Geometry: final body of the model. Coordinates: model frame, mm. Face numbers are marked on the shaded views. A direction names the side the tool comes from. Give positions to 0.01 mm unless a question says otherwise; leave off trailing zeros. Order: outer loops, then holes, each group sorted by start corner. A loop starts at its lowest first (then second) coordinate and runs counter-clockwise, first axis right, second up. Notation, with made-up numbers: (29.5, 49) - (73.5, 49) arc R17 cw to (73.5, 56) - close; hole circle Ø8 at (30, 88). An arc over 180 degrees is marked (long way). Put each result on its own line as item: value. Start each with the question number.
1. Ray query, line 1 along X through (y, z) = (-22, 3); line 2 along Y through (x, z) = (-36.5, 21); line 3 along X through (y, z) = (-43, 10). Return the intervals inside material, ascending. Write a range as from..to.
2. First-contact query: P1, Ø11, axis at y = -72, z = 28.5, coming from the +X side; P2, Ø1.5, axis at y = -9, z = 6, coming from the +X side; P3, Ø13.5, axis at x = -40, y = -15, coming from the +Z side. Flat tips, straight axial feed; report the tip coordinate or a pass-through.
3. Section B-B on x = -52.5. Return the cut outline in (y, z), plus the area to 3 significant figures.
4. Section D-D on y = -32.5. Return the cut outline in (x, z), plus the area to 3 significant figures.
5. Section C-C on z = 5. Return the cut outline in (x, y), plus the area to 3 significant figures.
6. Set-up query: the marked faces 1, 2 and 3. Return all of +Z, -Z, +X, -X, +Y, -Y with unobstructed straight access to the full face (end or side cutting, diameter ignored); none if empty.
7. Mould query, pull axis Y, two halves, no side actions, for the marked faces 4, 5 and 6. Classes: pulls with the +Y half, pulls with the -Y half, needs draft (parallel to the pull), parting line crosses it, or undercut.
8. Section A-A on z = 28. Return the cut outline in (x, y), plus the area to 3 significant figures.
from build123d import *

# Parameters (mm, degrees)
F0_W      = 100
F0_H      = 45
F1_DEPTH  = 80
F3_DEPTH  = 80
F5_DEPTH  = 20
F6_W      = 20
F6_H      = 15
F7_DEPTH  = 10
F8_R      = 7.5
F9_DEPTH  = 30
F11_DEPTH = 25


with BuildPart() as f1:
    # F0 (on Front) → F1 (new body)
    with BuildSketch(Plane.XZ):
        with Locations((-50, 22.5)):
            Rectangle(F0_W, F0_H)
    extrude(amount=F1_DEPTH)

    # F2 (on face) → F3 (cut, through all)
    with BuildSketch(Plane.XZ.offset(80)):
        with BuildLine():
            ThreePointArc((-16.3809735262, 45), (-4.2226032243, 23.944395449), (0, 0))
            Line((0, 0), (0, 45))
            Line((0, 45), (-16.3809735262, 45))
        make_face()
    extrude(amount=-F3_DEPTH, mode=Mode.SUBTRACT)

    # F4 (on face) → F5 (cut)
    with BuildSketch(Plane.XY.offset(45)):
        with BuildLine():
            Line((-100, -80), (-30, -80))
            ThreePointArc((-30, -80), (-50.5025253169, -30.5025253169), (-100, -10))
            Line((-100, -10), (-100, -80))
        make_face()
    extrude(amount=-F5_DEPTH, mode=Mode.SUBTRACT)

    # F6 (on face) → F7 (join)
    with BuildSketch(Plane.XY.offset(25)):
        with Locations((-90, -72.5)):
            Rectangle(F6_W, F6_H)
    extrude(amount=F7_DEPTH)

    # F8 (on face) → F9 (cut)
    with BuildSketch(Plane.XY.offset(45)):
        with Locations((-40, -15)):
            Circle(F8_R)
    extrude(amount=-F9_DEPTH, mode=Mode.SUBTRACT)

    # F10 (on face) → F11 (cut)
    with BuildSketch(Plane(origin=(0, 0, 0), x_dir=(1, 0, 0), z_dir=(0, 0, -1))):
        with BuildLine():
            Line((-36.7544467966, 50), (-65, 50))
            Line((-65, 50), (-65, 19.5))
            Line((-65, 19.5), (-64.7899162171, 19.5))
            ThreePointArc((-64.7899162171, 19.5), (-48.4641812562, 32.6284960508), (-36.7544467966, 50))
        make_face()
    extrude(amount=-F11_DEPTH, mode=Mode.SUBTRACT)


solid = f1.part
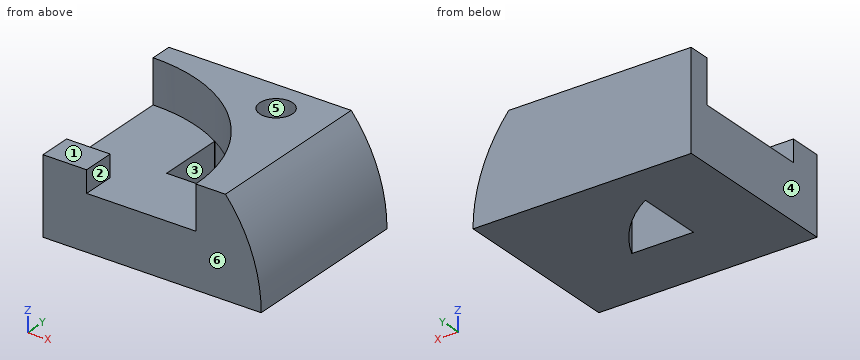
Resolved:
1. line 1: -100..-65, -60.81..-0.06
1. line 2: -80..-21.63, -8.37..0
1. line 3: -100..-65, -40.58..-0.72
2. P1: x = -3.89
2. P2: x = -0.2
2. P3: z = 15
3. outline: (-80, 0) - (-50, 0) - (-50, 25) - (-80, 25) - close; (-28.58, 0) - (0, 0) - (0, 45) - (-28.58, 45) - close
3. area: 2,040 mm^2
4. outline: (-100, 0) - (-65, 0) - (-65, 25) - (-100, 25) - close; (-48.58, 0) - (0, 0) arc R70 ccw to (-16.38, 45) - (-48.58, 45) - close
4. area: 2,830 mm^2
5. outline: (-100, -80) - (-0.18, -80) - (-0.18, 0) - (-100, 0) - close; hole (-65, -50) - (-36.75, -50) arc R70 ccw to (-64.79, -19.5) - (-65, -19.5) - close
5. area: 7,460 mm^2
6. face 1: +Z, -X, -Y
6. face 2: +Z, -Y
6. face 3: +Z, -Z
7. face 4: needs draft
7. face 5: undercut
7. face 6: pulls with the -Y half
8. outline: (-100, -80) - (-80, -80) - (-80, -65) - (-100, -65) - close; (-100, -10) arc R70 cw to (-30, -80) - (-5.84, -80) - (-5.84, 0) - (-100, 0) - close; hole circle Ø15 at (-40, -15)
8. area: 3,810 mm^2
